```python
from build123d import *

# Parameters (mm, degrees)
SKETCH2_R           = 1.715
SKETCH2_R_2         = 8.955
BOSS_EXTRUDE1_DEPTH = 2.5
BOSS_EXTRUDE2_START = 70.305
SKETCH3_R           = 1.715
SKETCH3_R_2         = 2.896004293
BOSS_EXTRUDE2_DEPTH = 70.305
BOSS_EXTRUDE3_START = 4
SKETCH4_R           = 21
SKETCH4_R_2         = 8.955
BOSS_EXTRUDE3_DEPTH = 4
CUT_EXTRUDE1_DEPTH  = 2
SKETCH6_R           = 21
SKETCH6_R_2         = 8.955
BOSS_EXTRUDE4_DEPTH = 2
CUT_EXTRUDE2_START  = -15
SKETCH7_R           = 1.715
CUT_EXTRUDE2_DEPTH  = 15


with BuildPart() as part:
    # Sketch2 → Boss-Extrude1 (new body)
    with BuildSketch(Plane(origin=(0, 0, 0), x_dir=(1, 0, 0), z_dir=(0, 1, 0))):
        with BuildLine():
            ThreePointArc((14.854844323, -2.224127391), (18.801958936, 0.560128045), (14.69610016, 3.104477828))
            ThreePointArc((14.69610016, 3.104477828), (9.742901135, 11.431929845), (0.735551003, 15.002403382))
            Line((0.735551003, 15.002403382), (0.735551003, 20.759778141))
            Line((0.735551003, 20.759778141), (-2.9930124, 20.759778141))
            Line((-2.9930124, 20.759778141), (-2.9930124, 14.719205797))
            ThreePointArc((-2.9930124, 14.719205797), (-10.557124207, 10.684580992), (-14.68222924, 3.169430082))
            ThreePointArc((-14.68222924, 3.169430082), (-18.635653921, 0.561038173), (-14.846301483, -2.280454949))
            ThreePointArc((-14.846301483, -2.280454949), (-10.873863647, -10.362057319), (-2.9930124, -14.719205797))
            Line((-2.9930124, -14.719205797), (-2.9930124, -17.45639334))
            Line((-2.9930124, -17.45639334), (0.735551003, -17.45639334))
            Line((0.735551003, -17.45639334), (0.735551003, -15.002403382))
            ThreePointArc((0.735551003, -15.002403382), (10.078997516, -11.136738821), (14.854844323, -2.224127391))
        make_face()
        with Locations(Location((15.90723889, 0.473891612, 0), (0, 0, 270))):
            Circle(SKETCH2_R, mode=Mode.SUBTRACT)
        with Locations(Location((-15.740961132, 0.473891612, 0), (0, 0, 270))):
            Circle(SKETCH2_R, mode=Mode.SUBTRACT)
        with Locations(Location((0, 0, 0), (0, 0, 270))):
            Circle(SKETCH2_R_2, mode=Mode.SUBTRACT)
    extrude(amount=-BOSS_EXTRUDE1_DEPTH)

    # Sketch3 → Boss-Extrude2 (add)
    # profile 1 of 3: a face of its own
    with BuildSketch(Plane(origin=(0, 0, 0), x_dir=(1, 0, 0), z_dir=(0, 1, 0)).offset(BOSS_EXTRUDE2_START)):
        with BuildLine():
            ThreePointArc((14.854844323, -2.224127391), (17.541114907, -1.917193921), (18.803243183, 0.473891612))
            ThreePointArc((18.803243183, 0.473891612), (17.469189258, 2.912569924), (14.69610016, 3.104477828))
            ThreePointArc((14.69610016, 3.104477828), (13.012518845, 0.387655178), (14.854844323, -2.224127391))
        make_face()
        with Locations(Location((15.90723889, 0.473891612, 0), (0, 0, 270))):
            Circle(SKETCH3_R, mode=Mode.SUBTRACT)
    # profile 2 of 3: a face of its own
    with BuildSketch(Plane(origin=(0, 0, 0), x_dir=(1, 0, 0), z_dir=(0, 1, 0)).offset(BOSS_EXTRUDE2_START)):
        with Locations(Location((15.90723889, 0.473891612, 0), (0, 0, 270))):
            Circle(SKETCH3_R)
    # profile 3 of 3: a face of its own
    with BuildSketch(Plane(origin=(0, 0, 0), x_dir=(1, 0, 0), z_dir=(0, 1, 0)).offset(BOSS_EXTRUDE2_START)):
        with Locations(Location((-15.740961132, 0.473891612, 0), (0, 0, 270))):
            Circle(SKETCH3_R_2)
    extrude(amount=-BOSS_EXTRUDE2_DEPTH)

    # Sketch4 → Boss-Extrude3 (add)
    with BuildSketch(Plane(origin=(0, 70.305, 0), x_dir=(1, 0, 0), z_dir=(0, 1, 0)).offset(BOSS_EXTRUDE3_START)):
        with Locations(Location((0, 0, 0), (0, 0, 270))):
            Circle(SKETCH4_R)
        with Locations(Location((0, 0, 0), (0, 0, 270))):
            Circle(SKETCH4_R_2, mode=Mode.SUBTRACT)
    extrude(amount=-BOSS_EXTRUDE3_DEPTH)

    # Sketch5 → Cut-Extrude1 (cut)
    with BuildSketch(Plane(origin=(0, 74.305, 0), x_dir=(1, 0, 0), z_dir=(0, 1, 0))):
        with BuildLine():
            Line((-7.35, 13.646519703), (-10, -0.003480297))
            Line((-10, -0.003480297), (-7.35, -13.653480297))
            ThreePointArc((-7.35, -13.653480297), (0, -15.506960594), (7.35, -13.653480297))
            Line((7.35, -13.653480297), (10, -0.003480297))
            Line((10, -0.003480297), (7.35, 13.646519703))
            ThreePointArc((7.35, 13.646519703), (0, 15.5), (-7.35, 13.646519703))
        make_face()
    extrude(amount=-CUT_EXTRUDE1_DEPTH, mode=Mode.SUBTRACT)

    # Sketch6 → Boss-Extrude4 (add)
    with BuildSketch(Plane(origin=(0, 35.305, 0), x_dir=(-1, 0, 0), z_dir=(0, -1, 0))):
        with Locations(Location((0, 0, 0), (0, 0, 270))):
            Circle(SKETCH6_R)
        with Locations(Location((0, 0, 0), (0, 0, 90))):
            Circle(SKETCH6_R_2, mode=Mode.SUBTRACT)
    extrude(amount=BOSS_EXTRUDE4_DEPTH)

    # Sketch7 → Cut-Extrude2 (cut)
    with BuildSketch(Plane.XZ.offset(2.5).offset(CUT_EXTRUDE2_START)):
        with Locations(Location((-15.740961132, -0.473891612, 0), (0, 0, 90))):
            Circle(SKETCH7_R)
        with Locations(Location((15.90723889, -0.473891612, 0), (0, 0, 90))):
            Circle(SKETCH7_R)
    extrude(amount=CUT_EXTRUDE2_DEPTH, mode=Mode.SUBTRACT)


solid = part.part
```
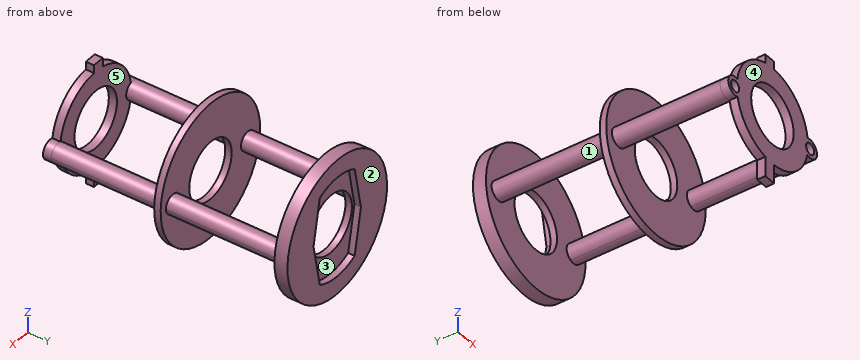
Geometry: final body of the model. Coordinates: model frame, mm. Face numbers are marked on the shaded views. A direction names the side the tool comes from. Round coordinates to 2 decimals unless told otherwise and drop trailing zeros. Order: outer loops, then holes, each group sorted by start corner. A loop starts at its lowest first (then second) coordinate and runs counter-clockwise, first axis right, second up. Notation, with made-up numbers: (-20, 46.25) - (-4, 46.25) arc R25 cw to (-4, 58.25) - close; hole circle Ø5 at (88.5, -32). An arc over 180 degrees is marked (long way). Write item = value, one per line. Start each with the question number.
Q1. Pin query (flat end, axial travel): pin 1 (23.5 mm diameter, centred on x = 0, z = 0, fed in from -Y); pin 2 (1 mm diameter, centred on x = -16.5, z = -1, fed in from -Y); pin 3 (3 mm diameter, centred on y = -1, z = -19, fed in from +X); pin 4 (5 mm diameter, centred on x = -6, y = 34, fed in from -Z). Return the tip coordinate at first contact, or that it passes through.
Q2. Cut plane B-B on y = 10. Return the cut outline in (x, z) (3 decimals).
Q3. Cut plane A-A on z = -7.5. Return the cut outline in (x, y) (3 decimals).
Q4. Pull-direction query (Y, two-part tool) for the marked faces 3, 4 and 5; classes: +Y half, -Y half, draft (parallel to the pull), parting line (faces both ways), or undercut.
Q5. Cut plane C-C on x = 3.5. Return the cut outline in (y, z) (3 decimals).
Q6. Access query for the marked faces 1 and 2. Directions: +Z, -Z, +X, -X, +Y, -Y. A direction counts if a zero-diameter tool reaches every point of the face in a straight line with its end or side. Return the directions, or none.
Q7. Ray query, line 1 (Y direction, x = -8, z = -9) (3 decimals); line 2 (Y direction, x = 9.5, z = -9.5) (3 decimals); line 3 (Y direction, x = 15, z = -14) (3 decimals). Return the intervals inside material, ascending. Write a range as from..to.
Q8. Cut plane D-D on y = 20.5. Return the cut outline in (x, z), and give its area (3 significant figures).
Outcome:
q1.pin_1 = -2.5
q1.pin_2 = 12.5
q1.pin_3 = 0.74
q1.pin_4 = -20.71
q2.outline = circle Ø5.792 at (-15.741, -0.474); circle Ø5.792 at (15.907, -0.474); hole circle Ø3.43 at (-15.741, -0.474); hole circle Ø3.43 at (15.907, -0.474)
q3.outline = (-19.615, 33.305) - (-4.893, 33.305) - (-4.893, 35.305) - (-19.615, 35.305) - close; (-19.615, 70.305) - (-4.893, 70.305) - (-4.893, 72.305) - (-8.543, 72.305) - (-8.543, 74.305) - (-19.615, 74.305) - close; (-13.014, -2.5) - (-4.893, -2.5) - (-4.893, 0) - (-13.014, 0) - close; (4.893, -2.5) - (13.014, -2.5) - (13.014, 0) - (4.893, 0) - close; (4.893, 33.305) - (19.615, 33.305) - (19.615, 35.305) - (4.893, 35.305) - close; (4.893, 70.305) - (19.615, 70.305) - (19.615, 74.305) - (8.543, 74.305) - (8.543, 72.305) - (4.893, 72.305) - close
q4.face_3 = +Y half
q4.face_4 = -Y half
q4.face_5 = undercut
q5.outline = (-2.5, -14.607) - (0, -14.607) - (0, -8.243) - (-2.5, -8.243) - close; (-2.5, 8.243) - (0, 8.243) - (0, 14.607) - (-2.5, 14.607) - close; (33.305, -20.706) - (35.305, -20.706) - (35.305, -8.243) - (33.305, -8.243) - close; (33.305, 8.243) - (35.305, 8.243) - (35.305, 20.706) - (33.305, 20.706) - close; (70.305, -20.706) - (74.305, -20.706) - (74.305, -15.1) - (72.305, -15.1) - (72.305, -8.243) - (70.305, -8.243) - close; (70.305, 8.243) - (72.305, 8.243) - (72.305, 15.107) - (74.305, 15.107) - (74.305, 20.706) - (70.305, 20.706) - close
q6.face_1 = none
q6.face_2 = +Z, -Z, +X, -X, +Y
q7.line_1 = -2.5..0, 33.305..35.305, 70.305..72.305
q7.line_2 = -2.5..0, 33.305..35.305, 70.305..74.305
q7.line_3 = 33.305..35.305, 70.305..74.305
q8.outline = circle Ø5.79 at (-15.74, -0.47); circle Ø5.79 at (15.91, -0.47)
q8.area = 52.7 mm^2
